```python
from build123d import *

# Parameters (mm, degrees)
ESQUISSE1_W             = 430
ESQUISSE1_H             = 180
BOSS_EXTRU_1_DEPTH      = 10
ESQUISSE2_W             = 80
ESQUISSE2_H             = 80
ENL_V_MAT_EXTRU_1_DEPTH = 10
ESQUISSE4_W             = 46
ESQUISSE4_H             = 11.2
ENL_V_MAT_EXTRU_2_DEPTH = 10


with BuildPart() as part:
    # Esquisse1 → Boss.-Extru.1 (new body)
    with BuildSketch(Plane.XY):
        with Locations((-215, 90)):
            Rectangle(ESQUISSE1_W, ESQUISSE1_H)
    extrude(amount=BOSS_EXTRU_1_DEPTH)

    # Esquisse2 → Enlèv. mat.-Extru.1 (cut)
    with BuildSketch(Plane(origin=(0, 0, 0), x_dir=(-1, 0, 0), z_dir=(0, 0, -1))):
        with Locations((80, 90)):
            Rectangle(ESQUISSE2_W, ESQUISSE2_H)
    extrude(amount=-ENL_V_MAT_EXTRU_1_DEPTH, mode=Mode.SUBTRACT)

    # Esquisse4 → Enlèv. mat.-Extru.2 (cut)
    with BuildSketch(Plane.XY.offset(10)):
        with Locations((-23, 5.6)):
            Rectangle(ESQUISSE4_W, ESQUISSE4_H)
        with Locations((-407, 5.6)):
            Rectangle(ESQUISSE4_W, ESQUISSE4_H)
    extrude(amount=-ENL_V_MAT_EXTRU_2_DEPTH, mode=Mode.SUBTRACT)


solid = part.part
```
Design review of the part built by this model. Coordinates are the model's own, in mm. A direction names the side the tool comes from. Coordinates: 2 decimals unless noted, no trailing zeros. Order: outer loops, then holes, each group sorted by start corner. A loop starts at its lowest first (then second) coordinate and runs counter-clockwise, first axis right, second up.
1) Take a section at C-C, the plane z = 3.75. Give the boundary of the cut face in (x, y).
2) Clearance check with flat-ended pins moving along their axes: pin 1 (2 mm diameter, centred on x = -234, y = 118.5, fed in from -Z); pin 2 (3 mm diameter, centred on x = -32, z = 5, fed in from -Y). State where each tip first meets the part, or that it passes through.
3) Take a section at A-A, the plane y = 55. Give the boundary of the cut face in (x, z), and give its area (3 significant figures).
4) For faces 1 (the flat face through (-46, 6, 5)), 2 (the flat face through (-407, 11.2, 5)), 3 (the flat face through (-218, 180, 5)), 4 (the flat face through (-120, 89, 5)), list the 3-axis set-ups (+Z, -Z, +X, -X, +Y, -Y) from which the entire face can be reached by the end or side of a thin tool; tool diameter is ignored.
5) Take a section at B-B, the plane x = -110. Give the boundary of the cut face in (y, z), and give its area (3 significant figures).
6) Mouldability with a two-part tool opening along X and no side actions: class faces 5 (the flat face through (-40, 89, 5)), 6 (the flat face through (-384, 6, 5)), 7 (the flat face through (-218, 91, 10)) as +X half, -X half, draft (parallel to the pull), parting line (faces both ways), or undercut.
7) Wall thickness on line 1 along X through (y, z) = (101.5, 4.75); line 2 along Y through (x, z) = (-52, 5.25); line 3 along Y through (x, z) = (-392.5, 9): over which ranges is each line inside the solid? List them lowest first.
Returned:
1. outline: (-430, 11.2) - (-384, 11.2) - (-384, 0) - (-46, 0) - (-46, 11.2) - (0, 11.2) - (0, 180) - (-430, 180) - close; hole (-120, 50) - (-40, 50) - (-40, 130) - (-120, 130) - close
2. pin 1: stops at z = 0
2. pin 2: stops at y = 11.2
3. outline: (-430, 0) - (-120, 0) - (-120, 10) - (-430, 10) - close; (-40, 0) - (0, 0) - (0, 10) - (-40, 10) - close
3. area: 3,500 mm2
4. face 1: +Z, -Z, +X, -Y
4. face 2: +Z, -Z, -X, -Y
4. face 3: +Z, -Z, +X, -X, +Y
4. face 4: +Z, -Z
5. outline: (0, 0) - (50, 0) - (50, 10) - (0, 10) - close; (130, 0) - (180, 0) - (180, 10) - (130, 10) - close
5. area: 1,000 mm2
6. face 5: undercut
6. face 6: -X half
6. face 7: draft
7. line 1: x = -430 to -120, -40 to 0
7. line 2: y = 0 to 50, 130 to 180
7. line 3: y = 11.2 to 180
